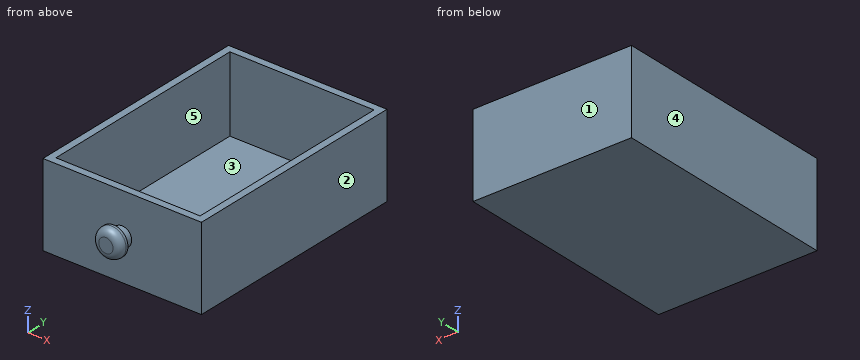
from build123d import *

# Parameters (mm, degrees)
F0_W     = 385.318
F0_H     = 201.168
F1_DEPTH = 19.05
F0_W_2   = 19.05
F0_H_2   = 19.05
F2_DEPTH = 590.55
F3_W     = 423.418
F3_H     = 220.218
F4_DEPTH = 19.05
F5_R     = 25.4
F6_DEPTH = 25.4
F8_R     = 38.1
F9_DEPTH = 25.4
F10_R    = 19.05


with BuildPart() as f1:
    # F0 (on Front) → F1 (new body)
    with BuildSketch(Plane.XZ):
        with Locations((2.090853, 45.724981)):
            Rectangle(F0_W, F0_H)
    extrude(amount=F1_DEPTH)

    # F0 (on Front) → F2 (join)
    with BuildSketch(Plane.XZ):
        with Locations((204.274853, 45.724981)):
            Rectangle(F0_W_2, F0_H)
        with Locations((-200.093147, 45.724981)):
            Rectangle(F0_W_2, F0_H)
        with Locations((2.090853, -64.384019)):
            Rectangle(F0_W, F0_H_2)
        with Locations((-200.093147, -64.384019)):
            Rectangle(F0_W_2, F0_H_2)
        with Locations((204.274853, -64.384019)):
            Rectangle(F0_W_2, F0_H_2)
    extrude(amount=F2_DEPTH)

    # F3 (on face) → F4 (join)
    with BuildSketch(Plane.XZ.offset(590.55)):
        with Locations((2.090853, 36.199981)):
            Rectangle(F3_W, F3_H)
    extrude(amount=F4_DEPTH)

    # F5 (on face) → F6 (join)
    with BuildSketch(Plane.XZ.offset(609.6)):
        with Locations((1.963853, 36.326981)):
            Circle(F5_R)
    extrude(amount=F6_DEPTH)

    # F8 (on face) → F9 (join)
    with BuildSketch(Plane.XZ.offset(635)):
        with Locations((0, 36.326981)):
            Circle(F8_R)
    extrude(amount=F9_DEPTH)

    # F10
    f10_edges = [f1.edges().sort_by_distance(p)[0] for p in [
        (-38.1, -660.4, 36.326981),
    ]]
    fillet(f10_edges, radius=F10_R)


solid = f1.part
Read the model definition and answer for the solid it produces. Units are mm, in the model's axes. Face numbers are marked on the shaded views. A direction names the side the tool comes from. Coordinates: 2 decimals unless noted, no trailing zeros. Loops run counter-clockwise (first coordinate to the right, second up) from the corner with the lowest first, then second, coordinate; pieces in that order, holes last. Notation, with made-up numbers: (-36, 18) -> (-15, 18) arc R20 cw to (-15, 45) -> close; hole circle Ø3 at (-13, -1.5). An arc over 180 degrees is marked (long way). Write item = value, one per line. Start each with the question number.
1) The part is cut by section C-C, the plane y = -229. Determine the outline of the cut face in (x, z), plus the area to 3 significant figures.
2) The mould has two halves that part along Y. Classify the marked faces 1, 2 and 3: pulls with the +Y half, pulls with the -Y half, needs draft (parallel to the pull), parting line crosses it, or undercut.
3) The part is cut by section A-A, the plane z = -19. Determine the outline of the cut face in (x, y).
4) The part is cut by section B-B, the plane x = 98. Determine the outline of the cut face in (y, z).
5) Given P1, Ø3, axis at x = 56.5, z = -35, coming from the -Y side; P2, Ø1, axis at x = 15.5, y = -578.5, coming from the +Z side, each flat-ended and moving along its own axis, determine where each tip first touches the part or whether it passes through.
6) Find the intervals of material crossed by L1, parallel to X at y = -531, z = 44; L2, parallel to Y at x = -41, z = 126; L3, parallel to Z at x = -163.5, y = -328.5, in increasing order. Write a range as from..to.
7) For the marked faces 4 and 5, determine the directions among +Z, -Z, +X, -X, +Y, -Y from which every point of the face is accessible in a straight line to the end or side of a thin tool.
Result:
q1.outline = (-209.62, -73.91) -> (213.8, -73.91) -> (213.8, 146.31) -> (194.75, 146.31) -> (194.75, -54.86) -> (-190.57, -54.86) -> (-190.57, 146.31) -> (-209.62, 146.31) -> close
q1.area = 15,700 mm²
q2.face_1 = pulls with the +Y half
q2.face_2 = needs draft
q2.face_3 = undercut
q3.outline = (-209.62, -609.6) -> (213.8, -609.6) -> (213.8, 0) -> (-209.62, 0) -> close; hole (-190.57, -590.55) -> (194.75, -590.55) -> (194.75, -19.05) -> (-190.57, -19.05) -> close
q4.outline = (-609.6, -73.91) -> (0, -73.91) -> (0, 146.31) -> (-19.05, 146.31) -> (-19.05, -54.86) -> (-590.55, -54.86) -> (-590.55, 146.31) -> (-609.6, 146.31) -> close
q5.P1 = -609.6
q5.P2 = -54.86
q6.L1 = -209.62..-190.57, 194.75..213.8
q6.L2 = -609.6..-590.55, -19.05..0
q6.L3 = -73.91..-54.86
q7.face_4 = +Z, -Z, -X, +Y, -Y
q7.face_5 = +Z
